Verification items for the finished model (mm, model axes). A direction names the side the tool comes from. Give positions to 0.01 mm unless a question says otherwise; leave off trailing zeros. Loops run counter-clockwise (first coordinate to the right, second up) from the corner with the lowest first, then second, coordinate; pieces in that order, holes last. Notation, with made-up numbers: (64, 79.5) - (89, 79.5) arc R34 ccw to (89, 109.5) - close; hole circle Ø7 at (49.25, 50.25). An arc over 180 degrees is marked (long way). One line per question, with ' | ' between items. Start each with the question number.
1. Tool access check on faces 4 (the face through (2.5, 9, 0)), 5 (the face through (3, 1, -50.5)), 6 (the face through (0, 8, -35.5)). Record the directions out of +Z, -Z, +X, -X, +Y, -Y that give a thin tool (end or side, any length) a straight path to the whole face; none if there is none.
2. Section check A-A, the plane y = 0. Enter the section's corners in (x, z), then the cut area to 3 significant figures.
3. Thickness scan on line 1 along Y through (x, z) = (0.5, -5); line 2 along X through (y, z) = (0, -47.25); line 3 along X through (y, z) = (0, -29). Record the ranges inside material, lowest first. Write a range as from..to.
4. Section check B-B, the plane z = 2.5. Enter the section's corners in (x, y).
5. Section check D-D, the plane x = 7. Enter the section's corners in (y, z).
6. Depth check by flat-ended pin: pin 1 Ø10 at (x, z) = (-9, -44) entering from +Y; pin 2 Ø1 at (x, z) = (1.5, -26.5) entering from +Y; pin 3 Ø6 at (y, z) = (13.5, -19) entering from -X. Enter the tip coordinate at first touch or a pass-through.
7. Mould release check, pull along Y, two halves, no side actions. Record for faces 1 (the face through (-1.38, 6.2, -42.9)), 2 (the face through (0, -8, 0)), 3 (the face through (4, -8, 10.5)): +Y half, -Y half, draft (parallel to the pull), parting line (faces both ways), or undercut.
8. Section check C-C, the plane x = 0. Enter the section's corners in (y, z), then the cut area to 3 significant figures.
from build123d import *

# Parameters (mm, degrees)
F0_R     = 17.5
F1_DEPTH = 10.5
F2_R     = 17.5
F2_R_2   = 2.75
F3_DEPTH = 25
F4_R     = 6.35
F4_R_2   = 2.75
F5_DEPTH = 15


with BuildPart() as f1:
    # F0 (on Top) → F1 (new body, symmetric)
    with BuildSketch(Plane.XY):
        Circle(F0_R)
        with BuildLine():
            ThreePointArc((2.5, 7.5993420768), (0, -8), (-2.5, 7.5993420768))
            Line((-2.5, 7.5993420768), (-2.5, 10))
            Line((-2.5, 10), (2.5, 10))
            Line((2.5, 10), (2.5, 7.5993420768))
        make_face(mode=Mode.SUBTRACT)
    extrude(amount=F1_DEPTH, both=True)

    # F2 (on face) → F3 (join)
    with BuildSketch(Plane(origin=(0, 0, -10.5), x_dir=(1, 0, 0), z_dir=(0, 0, -1))):
        Circle(F2_R)
        with BuildLine():
            Line((-2.5, -10), (-2.5, -7.5993420768))
            ThreePointArc((-2.5, -7.5993420768), (0, 8), (2.5, -7.5993420768))
            Line((2.5, -7.5993420768), (2.5, -10))
            Line((2.5, -10), (-2.5, -10))
        make_face(mode=Mode.SUBTRACT)
        with BuildLine():
            ThreePointArc((2.5, -7.5993420768), (0, 8), (-2.5, -7.5993420768))
            Line((-2.5, -7.5993420768), (-2.5, -10))
            Line((-2.5, -10), (2.5, -10))
            Line((2.5, -10), (2.5, -7.5993420768))
        make_face()
        Circle(F2_R_2, mode=Mode.SUBTRACT)
    extrude(amount=F3_DEPTH)

    # F4 (on face) → F5 (join)
    with BuildSketch(Plane(origin=(0, 0, -35.5), x_dir=(1, 0, 0), z_dir=(0, 0, -1))):
        Circle(F4_R)
        Circle(F4_R_2, mode=Mode.SUBTRACT)
    extrude(amount=F5_DEPTH)


solid = f1.part
Results list:
1) face 4: +Z | face 5: -Z, +X, -X, +Y, -Y | face 6: -Z
2) outline: (-17.5, -35.5) - (-6.35, -35.5) - (-6.35, -50.5) - (-2.75, -50.5) - (-2.75, -10.5) - (-8, -10.5) - (-8, 10.5) - (-17.5, 10.5) - close; (2.75, -50.5) - (6.35, -50.5) - (6.35, -35.5) - (17.5, -35.5) - (17.5, 10.5) - (8, 10.5) - (8, -10.5) - (2.75, -10.5) - close | area: 1,240 mm²
3) line 1: -17.49..-7.98, 10..17.49 | line 2: -6.35..-2.75, 2.75..6.35 | line 3: -17.5..-2.75, 2.75..17.5
4) outline: circle Ø35 at (0, 0); hole (-2.5, 7.6) arc R8 ccw (long way) to (2.5, 7.6) - (2.5, 10) - (-2.5, 10) - close
5) outline: (-16.04, -35.5) - (16.04, -35.5) - (16.04, 10.5) - (3.87, 10.5) - (3.87, -10.5) - (-3.87, -10.5) - (-3.87, 10.5) - (-16.04, 10.5) - close
6) pin 1: y = 4.93 | pin 2: y = 17.47 | pin 3: x = -14
7) face 1: parting line | face 2: undercut | face 3: draft
8) outline: (-17.5, -35.5) - (-6.35, -35.5) - (-6.35, -50.5) - (-2.75, -50.5) - (-2.75, -10.5) - (-8, -10.5) - (-8, 10.5) - (-17.5, 10.5) - close; (2.75, -50.5) - (6.35, -50.5) - (6.35, -35.5) - (17.5, -35.5) - (17.5, 10.5) - (10, 10.5) - (10, -10.5) - (2.75, -10.5) - close | area: 1,200 mm²
